```python
from build123d import *

# Parameters (mm, degrees)
F0_R     = 5.55625
F1_DEPTH = 0.79375
F2_R     = 2.38125
F3_DEPTH = 25.4
F4_R     = 0.254
F5_R     = 0.254


with BuildPart() as f1:
    # F0 (on Front) → F1 (new body, symmetric)
    with BuildSketch(Plane.XZ):
        Circle(F0_R)
    extrude(amount=F1_DEPTH, both=True)

    # F2 (on Front) → F3 (cut, symmetric)
    with BuildSketch(Plane.XZ):
        Circle(F2_R)
    extrude(amount=F3_DEPTH, both=True, mode=Mode.SUBTRACT)

    # F4
    f4_edges = [f1.edges().sort_by_distance(p)[0] for p in [
        (-2.38125, 0.79375, 0),
    ]]
    fillet(f4_edges, radius=F4_R)

    # F5
    f5_edges = [f1.edges().sort_by_distance(p)[0] for p in [
        (-5.55625, 0.79375, 0),
    ]]
    fillet(f5_edges, radius=F5_R)


solid = f1.part
```
Design review of the part built by this model. Coordinates are the model's own, in mm. Round coordinates to 2 decimals unless told otherwise and drop trailing zeros. Write each loop counter-clockwise with the first axis right and the second up, starting at its lowest first coordinate (ties: lowest second). Pieces come first, ordered by that corner, then holes. Notation, with made-up numbers: (39.25, -3) -> (75.25, -3) arc R13 ccw to (75.25, 5) -> close; hole circle Ø10 at (38, 75). An arc over 180 degrees is marked (long way). Answer in a Markdown table with one row per item.
Q1. To check wall thickness, follow L1, parallel to Z at x = 0, y = -0.1; L2, parallel to X at y = -0.45, z = 1.25; L3, parallel to Z at x = 1.75, y = -0.3. State the ranges of each line that lie inside material, in increasing order. Write a range as [from, to].
The answers:
| item | result |
|---|---|
| L1 | [-5.56, -2.38], [2.38, 5.56] |
| L2 | [-5.41, -2.03], [2.03, 5.41] |
| L3 | [-5.27, -1.61], [1.61, 5.27] |
Q2. Take a section at A-A, the plane x = 0. State the section outline as (y, z) points.
The answers:
| item | result |
|---|---|
| outline | (-0.79, -5.56) -> (0.54, -5.56) arc R0.25 ccw to (0.79, -5.3) -> (0.79, -2.64) arc R0.25 ccw to (0.54, -2.38) -> (-0.79, -2.38) -> close; (-0.79, 2.38) -> (0.54, 2.38) arc R0.25 ccw to (0.79, 2.64) -> (0.79, 5.3) arc R0.25 ccw to (0.54, 5.56) -> (-0.79, 5.56) -> close |
Q3. Clearance check with flat-ended pins moving along their axes: pin 1 Ø4 at (x, z) = (0, 0) entering from -Y; pin 2 Ø2 at (x, z) = (-1.5, -0.5) entering from +Y. State where each tip first meets the part, or that it passes through.
The answers:
| item | result |
|---|---|
| pin 1 | through |
| pin 2 | y = 0.79 |
Q4. Take a section at B-B, the plane y = -0.15. State the section outline as (x, z) points, then the cut area to 3 significant figures.
The answers:
| item | result |
|---|---|
| outline | circle Ø11.11 at (0, 0); hole circle Ø4.76 at (0, 0) |
| area | 79.2 mm² |
